Check sheet for the modelled part. Datum: model origin and axes. Units: mm. A direction names the side the tool comes from. Give positions to 0.01 mm unless a question says otherwise; leave off trailing zeros. Write each loop counter-clockwise with the first axis right and the second up, starting at its lowest first coordinate (ties: lowest second). Pieces come first, ordered by that corner, then holes. Notation, with made-up numbers: (-7.5, 19) -> (24.5, 19) arc R29 ccw to (24.5, 53) -> close; hole circle Ø4 at (62, 25.5). An arc over 180 degrees is marked (long way). Write each question's results on one line, items separated by ' | '. Start each with the question number.
```python
from build123d import *

# Parameters (mm, degrees)
SKETCH_1_W               = 31.8
SKETCH_1_H               = 26.8
SKETCH_1_R               = 1
EXTRUDE_1_DEPTH          = 1.6
EXTRUDE_2_DEPTH          = 4
SKETCH_2_W               = 5.4
SKETCH_2_H               = 16
CUT_EXTRUDE_1_DEPTH      = 0.8
EXTRUDE_3_DEPTH          = 33.8
SKETCH_4_R               = 1.6
CUT_EXTRUDE_2_DEPTH      = 31.944627967
CUT_EXTRUDE_2_DEPTH_BACK = 31.944627967
CUT_EXTRUDE_START        = -1
SKETCH_6_R               = 3.2
SKETCH_6_R_2             = 1.6
CUT_EXTRUDE_3_DEPTH      = 3
CUT_EXTRUDE_START_2      = 1.6
SKETCH_1_5_R             = 1
CUT_EXTRUDE_5_DEPTH      = 33.544628089
FILLET_1_R               = 1
SKETCH_7_R               = 1.5
SKETCH_7_R_2             = 1
CUT_EXTRUDE_6_DEPTH      = 0.8


with BuildPart() as part:
    # Эскиз1 → Бобышка-Вытянуть1 (new body)
    with BuildSketch(Plane.XY):
        Rectangle(SKETCH_1_W, SKETCH_1_H)
        with Locations((-8.5, -11)):
            Circle(SKETCH_1_R, mode=Mode.SUBTRACT)
        with Locations((-8.5, 11)):
            Circle(SKETCH_1_R, mode=Mode.SUBTRACT)
        with Locations((13.5, 11)):
            Circle(SKETCH_1_R, mode=Mode.SUBTRACT)
        with Locations((13.5, -11)):
            Circle(SKETCH_1_R, mode=Mode.SUBTRACT)
        with Locations((-8.5, 11)):
            Circle(SKETCH_1_R)
        with Locations((13.5, 11)):
            Circle(SKETCH_1_R)
        with Locations((-8.5, -11)):
            Circle(SKETCH_1_R)
        with Locations((13.5, -11)):
            Circle(SKETCH_1_R)
    extrude(amount=EXTRUDE_1_DEPTH)

    # Эскиз1<3> → Бобышка-Вытянуть2 (add)
    with BuildSketch(Plane.XY):
        Polygon((-15.9, -13.4), (-15.9, -15.4), (17.9, -15.4), (17.9, 15.4), (-15.9, 15.4), (-15.9, 13.4), (15.9, 13.4), (15.9, -13.4), align=None)
    extrude(amount=EXTRUDE_2_DEPTH)

    # Эскиз2 → Вырез-Вытянуть1 (cut)
    with BuildSketch(Plane.XY.offset(1.6)):
        with Locations((13.2, 0)):
            Rectangle(SKETCH_2_W, SKETCH_2_H)
    extrude(amount=-CUT_EXTRUDE_1_DEPTH, mode=Mode.SUBTRACT)

    # Эскиз3 → Бобышка-Вытянуть3 (add)
    with BuildSketch(Plane.ZY.offset(15.9)):
        with BuildLine():
            Line((-1.6, 0), (0, 0))
            ThreePointArc((0, 0), (-2.928932188, 7.071067812), (-10, 10))
            ThreePointArc((-10, 10), (-17.071067812, 7.071067812), (-20, 0))
            Line((-20, 0), (-18.4, 0))
            ThreePointArc((-18.4, 0), (-10, 8.4), (-1.6, 0))
        make_face()
        with BuildLine():
            ThreePointArc((-10, -10), (-2.928932188, -7.071067812), (0, 0))
            Line((0, 0), (-1.6, 0))
            ThreePointArc((-1.6, 0), (-10, -8.4), (-18.4, 0))
            Line((-18.4, 0), (-20, 0))
            ThreePointArc((-20, 0), (-17.071067812, -7.071067812), (-10, -10))
        make_face()
        with BuildLine():
            Line((0, -10), (0, 0))
            ThreePointArc((0, 0), (-2.928932188, -7.071067812), (-10, -10))
            Line((-10, -10), (0, -10))
        make_face()
        with BuildLine():
            ThreePointArc((-10, 10), (-2.928932188, 7.071067812), (0, 0))
            Line((0, 0), (0, 10))
            Line((0, 10), (-10, 10))
        make_face()
    extrude(amount=-EXTRUDE_3_DEPTH)

    # Эскиз4 → Вырез-Вытянуть2 (cut, two sides)
    with BuildSketch(Plane(origin=(0, 0, 0), x_dir=(1, 0, 0), z_dir=(0, 1, 0))) as cut_extrude_2_sk:
        with Locations(Location((-7.9, 10, 0), (0, 0, 270))):
            Circle(SKETCH_4_R)
        with Locations(Location((7.9, 10, 0), (0, 0, 270))):
            Circle(SKETCH_4_R)
    extrude(amount=CUT_EXTRUDE_2_DEPTH, mode=Mode.SUBTRACT)
    extrude(cut_extrude_2_sk.sketch, amount=-CUT_EXTRUDE_2_DEPTH_BACK, mode=Mode.SUBTRACT)

    # Эскиз6 → Вырез-Вытянуть3 (cut)
    with BuildSketch(Plane(origin=(0, 10.08, 0), x_dir=(1, 0, 0), z_dir=(0, 1, 0)).offset(CUT_EXTRUDE_START)):
        with Locations((7.9, 10)):
            Circle(SKETCH_6_R)
        with Locations(Location((7.9, 10, 0), (0, 0, 270))):
            Circle(SKETCH_6_R_2, mode=Mode.SUBTRACT)
        with Locations((-7.9, 10)):
            Circle(SKETCH_6_R)
        with Locations(Location((-7.9, 10, 0), (0, 0, 270))):
            Circle(SKETCH_6_R_2, mode=Mode.SUBTRACT)
    cut_extrude_3 = extrude(amount=CUT_EXTRUDE_3_DEPTH, mode=Mode.SUBTRACT)

    # Зеркальное отражение1: Вырез-Вытянуть3 across plane
    add(cut_extrude_3.mirror(Plane.ZX), mode=Mode.SUBTRACT)

    # Эскиз1<5> → Вырез-Вытянуть5 (cut, through all)
    with BuildSketch(Plane.XY.offset(CUT_EXTRUDE_START_2)):
        with Locations((13.5, 11)):
            Circle(SKETCH_1_5_R)
        with Locations((-8.5, 11)):
            Circle(SKETCH_1_5_R)
        with Locations((-8.5, -11)):
            Circle(SKETCH_1_5_R)
        with Locations((13.5, -11)):
            Circle(SKETCH_1_5_R)
    extrude(amount=-CUT_EXTRUDE_5_DEPTH, mode=Mode.SUBTRACT)

    # Скругление1
    fillet_1_edges = [part.edges().sort_by_distance(p)[0] for p in [
        (1, -15.4, 0),
        (1, 15.4, 4),
        (1, -15.4, 4),
        (1, 15.4, 0),
    ]]
    fillet(fillet_1_edges, radius=FILLET_1_R)

    # Эскиз7 → Вырез-Вытянуть6 (cut)
    with BuildSketch(Plane(origin=(0, 0, 0), x_dir=(-1, 0, 0), z_dir=(0, 0, -1))):
        with Locations((8.5, 11)):
            Circle(SKETCH_7_R)
        with Locations(Location((8.5, 11, 0), (0, 0, 180))):
            Circle(SKETCH_7_R_2, mode=Mode.SUBTRACT)
        with Locations((-13.5, 11)):
            Circle(SKETCH_7_R)
        with Locations(Location((-13.5, 11, 0), (0, 0, 180))):
            Circle(SKETCH_7_R_2, mode=Mode.SUBTRACT)
        with Locations((8.5, -11)):
            Circle(SKETCH_7_R)
        with Locations(Location((8.5, -11, 0), (0, 0, 180))):
            Circle(SKETCH_7_R_2, mode=Mode.SUBTRACT)
        with Locations((-13.5, -11)):
            Circle(SKETCH_7_R)
        with Locations(Location((-13.5, -11, 0), (0, 0, 180))):
            Circle(SKETCH_7_R_2, mode=Mode.SUBTRACT)
    extrude(amount=CUT_EXTRUDE_6_DEPTH, mode=Mode.SUBTRACT)


solid = part.part
```
Item 1: Thickness scan on probe 1 along Y at (x, z) = (1, -10); probe 2 along Y at (x, z) = (13.5, 1.05); probe 3 along Y at (x, z) = (8.5, 2.25). Record the ranges inside material, lowest first. Write a range as from..to.
Item 2: Section check B-B on y = -11. Record the boundary of the cut face in (x, z).
Item 3: Mould release check, pull along Y, two halves, no side actions. Record for faces 4 (the flat face through (6, -9.08, -9)), 5 (the flat face through (-6.5, 9.08, -8.6)), 6 (the flat face through (0, 13.4, 3)): pulls with the +Y half, pulls with the -Y half, needs draft (parallel to the pull), parting line crosses it, or undercut.
Item 4: Section check C-C on z = -16.25. Record the boundary of the cut face in (x, y).
Item 5: Set-up check for faces 1 (the cylindrical face through (-8.594, -9.534, -6.876)), 2 (the flat face through (13, 0, 0.8)), 3 (the flat face through (1, -10, -5)): record each of +Z, -Z, +X, -X, +Y, -Y from which the full face is reachable in a straight line by a thin tool's end or side.
Item 6: Section check A-A on x = 13.5. Count the separate pieces of the cut face and the enclosed holes in it, then the cut area to 3 significant figures.
Item 7: Depth check by flat-ended pin: pin 1 Ø1.8 at (x, y) = (13.5, -11) entering from -Z; pin 2 Ø3 at (x, z) = (9, -8.5) entering from +Y; pin 3 Ø4 at (x, z) = (1.5, -7) entering from -Y; pin 4 Ø0.6 at (x, y) = (14, 10) entering from +Z. Enter the tip coordinate at first touch or a pass-through.
Item 8: Section check D-D on x = 3. Record the boundary of the cut face in (y, z).
Check sheet entries:
1) probe 1: y = -10..-8.4, 8.4..10 | probe 2: y = -15.4..-12, -10..-8, 8..10, 12..15.4 | probe 3: y = -15.4..-13.4, 13.4..15.4
2) outline: (-15.9, 0) -> (-9.5, 0) -> (-9.5, 1.6) -> (-15.9, 1.6) -> close; (-7.5, 0) -> (12.5, 0) -> (12.5, 1.6) -> (-7.5, 1.6) -> close; (14.5, 0) -> (17.9, 0) -> (17.9, 4) -> (15.9, 4) -> (15.9, 1.6) -> (14.5, 1.6) -> close
3) face 4: pulls with the -Y half | face 5: pulls with the +Y half | face 6: undercut
4) outline: (-15.9, -7.81) -> (17.9, -7.81) -> (17.9, -5.61) -> (-15.9, -5.61) -> close; (-15.9, 5.61) -> (17.9, 5.61) -> (17.9, 7.81) -> (-15.9, 7.81) -> close
5) face 1: -Y | face 2: +Z | face 3: -Z, +X, -X, -Y
6) separate pieces: 3 | enclosed holes: 1 | area: 173 mm^2
7) pin 1: passes through | pin 2: stops at y = 10 | pin 3: stops at y = -10 | pin 4: stops at z = 1.6
8) outline: (-15.4, 1) arc R1 ccw to (-14.4, 0) -> (-10, 0) -> (-10, -10) arc R10 ccw to (10, -10) -> (10, 0) -> (14.4, 0) arc R1 ccw to (15.4, 1) -> (15.4, 3) arc R1 ccw to (14.4, 4) -> (13.4, 4) -> (13.4, 1.6) -> (-13.4, 1.6) -> (-13.4, 4) -> (-14.4, 4) arc R1 ccw to (-15.4, 3) -> close; hole circle Ø16.8 at (0, -10)
